Geometry check sheet. Reference: the model listing, model coordinates, mm. Give positions to 0.01 mm unless a question says otherwise; leave off trailing zeros. Loops run counter-clockwise (first coordinate to the right, second up) from the corner with the lowest first, then second, coordinate; pieces in that order, holes last. Notation, with made-up numbers: (87, -16) -> (121, -16) arc R24 ccw to (121, 1) -> close; hole circle Ø9 at (-17.5, -34.5). An arc over 180 degrees is marked (long way). Answer as a JSON object with one key per item and string values.
Autodesk Inventor part; units mm, degrees
ref_plane "YZ Plane" through (0, 0, 0) normal (1, 0, 0) x (0, 1, 0)
ref_plane "XZ Plane" through (0, 0, 0) normal (0, 1, 0) x (-1, 0, 0)
ref_plane "XY Plane" through (0, 0, 0) normal (0, 0, 1) x (1, 0, 0)
sketch "Sketch1" plane through (0, 0, 0) normal (0, 0, 1) x (1, 0, 0)
  line L0 (0, 0) -> (247.65, 0)
  line L1 (762, 0) -> (762, 368.3)
  line L2 (762, 368.3) -> (0, 368.3)
  line L3 (0, 368.3) -> (0, 0)
  line L4 (752.475, 368.3) -> (752.475, 0) construction
  line L5 (762, 184.15) -> (0, 184.15) construction
  line L6 (381, 368.3) -> (381, 0) construction
  line L7 (762, 238.125) -> (0, 238.125) construction
  circle A0 centre (381, 238.125) radius 1.5875
  circle A1 centre (295.275, 238.125) radius 1.5875
  circle A2 centre (209.55, 238.125) radius 1.5875
  circle A3 centre (123.825, 238.125) radius 1.5875
  circle A4 centre (38.1, 238.125) radius 1.5875
  circle A5 centre (466.725, 238.125) radius 1.5875
  circle A6 centre (552.45, 238.125) radius 1.5875
  circle A7 centre (638.175, 238.125) radius 1.5875
  circle A8 centre (723.9, 238.125) radius 1.5875
  circle A9 centre (752.475, 184.15) radius 1.5875
  circle A10 centre (752.475, 107.95) radius 1.5875
  circle A11 centre (752.475, 31.75) radius 1.5875
  circle A12 centre (752.475, 260.35) radius 1.5875
  circle A13 centre (752.475, 184.15) radius 1.5875
  circle A14 centre (752.475, 107.95) radius 1.5875
  circle A15 centre (752.475, 336.55) radius 1.5875
  circle A16 centre (752.475, 260.35) radius 1.5875
  circle A17 centre (752.475, 184.15) radius 1.5875
  line L8 (9.525, 368.3) -> (9.525, 0) construction
  circle A18 centre (9.525, 184.15) radius 1.5875
  circle A19 centre (9.525, 107.95) radius 1.5875
  circle A20 centre (9.525, 31.75) radius 1.5875
  circle A21 centre (9.525, 260.35) radius 1.5875
  circle A22 centre (9.525, 184.15) radius 1.5875
  circle A23 centre (9.525, 107.95) radius 1.5875
  circle A24 centre (9.525, 336.55) radius 1.5875
  circle A25 centre (9.525, 260.35) radius 1.5875
  circle A26 centre (9.525, 184.15) radius 1.5875
  line L9 (482.6, 0) -> (482.6, 228.6)
  line L10 (482.6, 228.6) -> (266.7, 228.6)
  line L11 (266.7, 228.6) -> (266.7, 50.8)
  line L12 (482.6, 0) -> (762, 0)
  line L13 (266.7, 0) -> (482.6, 0) construction
  line L14 (266.7, 50.8) -> (247.65, 50.8)
  line L15 (247.65, 50.8) -> (247.65, 0)
  line L16 (266.7, 50.8) -> (266.7, 0) construction
  line L17 (247.65, 0) -> (266.7, 0) construction
  dimension "d0" = 762
  dimension "d1" = 368.3
  dimension "d12" = 9.525
  dimension "d16" = 85.725
  dimension "d23" = 85.725
  dimension "d28" = 3.175
  dimension "d31" = 76.2
  dimension "d34" = 76.2
  dimension "d39" = 9.525
  dimension "d41" = 101.6
  dimension "d42" = 114.3
  dimension "d43" = 19.05
  dimension "d44" = 50.8
  dimension "d45" = 44.45
extrude "Extrusion1" add sketch "Sketch1" along normal blind 1.5875
properties part number "Long Wall" material "Polycarbonate, Clear"
1) Section check D-D on x = 254.5. Record the cut outline in (y, z), plus the area to 3 significant figures.
Geometry check:
{"outline": "(50.8, 0) -> (368.3, 0) -> (368.3, 1.59) -> (50.8, 1.59) -> close", "area": "504 mm2"}
2) Section check A-A on y = 217.5. Record the cut outline in (x, z).
Geometry check:
{"outline": "(0, 0) -> (266.7, 0) -> (266.7, 1.59) -> (0, 1.59) -> close; (482.6, 0) -> (762, 0) -> (762, 1.59) -> (482.6, 1.59) -> close"}
3) Section check B-B on z = 0.7. Count the separate pieces of the cut face and the enclosed holes in it, plus the area to 3 significant figures.
Geometry check:
{"separate pieces": "1", "enclosed holes": "19", "area": "230,000 mm2"}
4) Section check C-C on x = 342.5. Record the cut outline in (y, z).
Geometry check:
{"outline": "(228.6, 0) -> (368.3, 0) -> (368.3, 1.59) -> (228.6, 1.59) -> close"}
5) Material ranges on line 1 along X through (y, z) = (184.15, 1.15); line 2 along X through (y, z) = (260.35, 0.55); line 3 along X through (y, z) = (84.5, 1.1), recorded low to high. Write a range as from..to.
Geometry check:
{"line 1": "x = 0..7.94, 11.11..266.7, 482.6..750.89, 754.06..762", "line 2": "x = 0..7.94, 11.11..750.89, 754.06..762", "line 3": "x = 0..266.7, 482.6..762"}
6) Depth check by flat-ended pin: P1, Ø3, axis at x = 638.175, y = 238.125, coming from the -Z side; P2, Ø12, axis at x = 443.5, y = 303, coming from the -Z side. Enter the tip coordinate at first touch or a pass-through.
Geometry check:
{"P1": "passes through", "P2": "stops at z = 0"}
